from build123d import *

# Parameters (mm, degrees)
SKETCH1_W           = 15.8
SKETCH1_H           = 15.8
SKETCH1_W_2         = 13.8
SKETCH1_H_2         = 13.8
BOSS_EXTRUDE1_DEPTH = 150
SKETCH2_R           = 1.7
CUT_EXTRUDE1_DEPTH  = 152.036584972
SKETCH3_R           = 1.7
CUT_EXTRUDE3_DEPTH  = 152.036584972


with BuildPart() as part:
    # Sketch1 → Boss-Extrude1 (new body)
    with BuildSketch(Plane(origin=(0, 0, 0), x_dir=(1, 0, 0), z_dir=(0, 1, 0))):
        Rectangle(SKETCH1_W, SKETCH1_H)
        Rectangle(SKETCH1_W_2, SKETCH1_H_2, mode=Mode.SUBTRACT)
    extrude(amount=BOSS_EXTRUDE1_DEPTH)

    # Sketch2 → Cut-Extrude1 (cut, through all)
    with BuildSketch(Plane.ZY.offset(7.9)):
        with Locations((0, 115)):
            Circle(SKETCH2_R)
        with Locations(Location((0, 35, 0), (0, 0, 180))):
            Circle(SKETCH2_R)
    extrude(amount=-CUT_EXTRUDE1_DEPTH, mode=Mode.SUBTRACT)

    # Sketch3 → Cut-Extrude3 (cut, through all)
    with BuildSketch(Plane.XY.offset(7.9)):
        with Locations((0, 85)):
            Circle(SKETCH3_R)
        with Locations((0, 65)):
            Circle(SKETCH3_R)
    extrude(amount=-CUT_EXTRUDE3_DEPTH, mode=Mode.SUBTRACT)


solid = part.part
The model under review builds one solid part; all positions refer to its coordinate system, in mm. A direction names the side the tool comes from. Round coordinates to 2 decimals unless told otherwise and drop trailing zeros. Order: outer loops, then holes, each group sorted by start corner. A loop starts at its lowest first (then second) coordinate and runs counter-clockwise, first axis right, second up. Notation, with made-up numbers: (4, -7.5) -> (32, -7.5) arc R16 cw to (32, 2.5) -> close; hole circle Ø9 at (-25.75, 66). An arc over 180 degrees is marked (long way). Return JSON: item names as keys, results as strings.
1. Take a section at C-C (y = 35). Write out the cut boundary in (x, z), then the cut area to 3 significant figures.
Answer block:
{"outline": "(-7.9, -7.9) -> (7.9, -7.9) -> (7.9, -1.7) -> (6.9, -1.7) -> (6.9, -6.9) -> (-6.9, -6.9) -> (-6.9, -1.7) -> (-7.9, -1.7) -> close; (-7.9, 1.7) -> (-6.9, 1.7) -> (-6.9, 6.9) -> (6.9, 6.9) -> (6.9, 1.7) -> (7.9, 1.7) -> (7.9, 7.9) -> (-7.9, 7.9) -> close", "area": "52.4 mm²"}
2. Insertion check: P1, Ø2, axis at y = 115, z = 0, coming from the -X side. The pin has a flat end and moves straight along its axis. Give the tip position at first contact, or say it passes through.
Answer block:
{"P1": "passes through"}
3. For faces 1 (the face through (-7.9, 74, 0)), 2 (the face through (-6.9, 74, 0)), list the 3-axis set-ups (+Z, -Z, +X, -X, +Y, -Y) from which the entire face can be reached by the end or side of a thin tool; tool diameter is ignored.
Answer block:
{"face 1": "+Z, -Z, -X, +Y, -Y", "face 2": "+Y, -Y"}
4. Take a section at D-D (y = 100.5). Write out the cut boundary in (x, z), then the cut area to 3 significant figures.
Answer block:
{"outline": "(-7.9, -7.9) -> (7.9, -7.9) -> (7.9, 7.9) -> (-7.9, 7.9) -> close; hole (-6.9, -6.9) -> (6.9, -6.9) -> (6.9, 6.9) -> (-6.9, 6.9) -> close", "area": "59.2 mm²"}
5. Take a section at A-A (x = 0). Write out the cut boundary in (y, z), then the cut area to 3 significant figures.
Answer block:
{"outline": "(0, -7.9) -> (63.3, -7.9) -> (63.3, -6.9) -> (0, -6.9) -> close; (0, 6.9) -> (63.3, 6.9) -> (63.3, 7.9) -> (0, 7.9) -> close; (66.7, -7.9) -> (83.3, -7.9) -> (83.3, -6.9) -> (66.7, -6.9) -> close; (66.7, 6.9) -> (83.3, 6.9) -> (83.3, 7.9) -> (66.7, 7.9) -> close; (86.7, -7.9) -> (150, -7.9) -> (150, -6.9) -> (86.7, -6.9) -> close; (86.7, 6.9) -> (150, 6.9) -> (150, 7.9) -> (86.7, 7.9) -> close", "area": "286 mm²"}
6. Take a section at B-B (z = 0). Write out the cut boundary in (x, y).
Answer block:
{"outline": "(-7.9, 0) -> (-6.9, 0) -> (-6.9, 33.3) -> (-7.9, 33.3) -> close; (-7.9, 36.7) -> (-6.9, 36.7) -> (-6.9, 113.3) -> (-7.9, 113.3) -> close; (-7.9, 116.7) -> (-6.9, 116.7) -> (-6.9, 150) -> (-7.9, 150) -> close; (6.9, 0) -> (7.9, 0) -> (7.9, 33.3) -> (6.9, 33.3) -> close; (6.9, 36.7) -> (7.9, 36.7) -> (7.9, 113.3) -> (6.9, 113.3) -> close; (6.9, 116.7) -> (7.9, 116.7) -> (7.9, 150) -> (6.9, 150) -> close"}
7. The part is to be moulded in two halves that separate along Z. For faces 3 (the face through (0, 74, -7.9)), 4 (the face through (0, 74, 7.9)), 5 (the face through (-0.37, 83.34, -7.39)), 6 (the face through (0, 74, 6.9)), say which applies: +Z half, -Z half, draft (parallel to the pull), parting line (faces both ways), or undercut.
Answer block:
{"face 3": "-Z half", "face 4": "+Z half", "face 5": "draft", "face 6": "undercut"}
8. For L1, parallel to Y at x = 7.4, z = 0; L2, parallel to Y at x = 0, z = 7.5; L3, parallel to X at y = 144, z = -3.5, list the stretches that pass through material, from the lowest coordinate up. Write a range as [from, to].
Answer block:
{"L1": "y = [0, 33.3], [36.7, 113.3], [116.7, 150]", "L2": "y = [0, 63.3], [66.7, 83.3], [86.7, 150]", "L3": "x = [-7.9, -6.9], [6.9, 7.9]"}
